```python
from build123d import *

# Parameters (mm, degrees)
SKETCH2_R           = 4.5
BOSS_EXTRUDE1_DEPTH = 76
SKETCH3_W           = 19
SKETCH3_H           = 19
BOSS_EXTRUDE2_DEPTH = 6
CHAMFER1_SIZE       = 1
CHAMFER1_SIZE2      = 1.732050808
SKETCH4_OUTSIDE_W   = 50.258
SKETCH4_OUTSIDE_H   = 50.258
SKETCH4_OUTSIDE_R   = 9.5
CUT_EXTRUDE1_DEPTH  = 6
CUT_EXTRUDE1_DRAFT  = -45


with BuildPart() as part:
    # Sketch2 → Boss-Extrude1 (new body)
    with BuildSketch(Plane.XY):
        Circle(SKETCH2_R)
    extrude(amount=BOSS_EXTRUDE1_DEPTH)

    # Sketch3 → Boss-Extrude2 (add)
    with BuildSketch(Plane.XY.offset(76)):
        Rectangle(SKETCH3_W, SKETCH3_H)
    extrude(amount=BOSS_EXTRUDE2_DEPTH)

    # Chamfer1
    chamfer1_edges = [part.edges().sort_by_distance(p)[0] for p in [
        (-4.5, 0, 0),
    ]]
    chamfer1_side = [part.faces().sort_by_distance(p)[0] for p in [
        (0, 0, 0),
    ]]
    chamfer(chamfer1_edges, length=CHAMFER1_SIZE, length2=CHAMFER1_SIZE2, reference=chamfer1_side[0])


with BuildPart() as cut_extrude1_tool:
    # Sketch4 outside → Cut-Extrude1 (with draft: the straight prism first)
    with BuildSketch(Plane.XY.offset(82)):
        Rectangle(SKETCH4_OUTSIDE_W, SKETCH4_OUTSIDE_H)
        Circle(SKETCH4_OUTSIDE_R, mode=Mode.SUBTRACT)
    extrude(amount=-CUT_EXTRUDE1_DEPTH)
    # Cut-Extrude1: the draft: its side faces are tilted about the plane it starts from
    cut_extrude1_sides = [cut_extrude1_tool.faces().sort_by_distance(p)[0] for p in [
        (0, -25.129, 79),
        (25.129, 0, 79),
        (0, 25.129, 79),
        (-25.129, 0, 79),
        (-9.5, 0, 79),
    ]]
    draft(cut_extrude1_sides, Plane.XY.offset(82), CUT_EXTRUDE1_DRAFT)


with BuildPart() as part_1:
    add(part.part)

    # Cut-Extrude1: cut by cut_extrude1_tool
    add(cut_extrude1_tool.part, mode=Mode.SUBTRACT)


solid = part_1.part
```
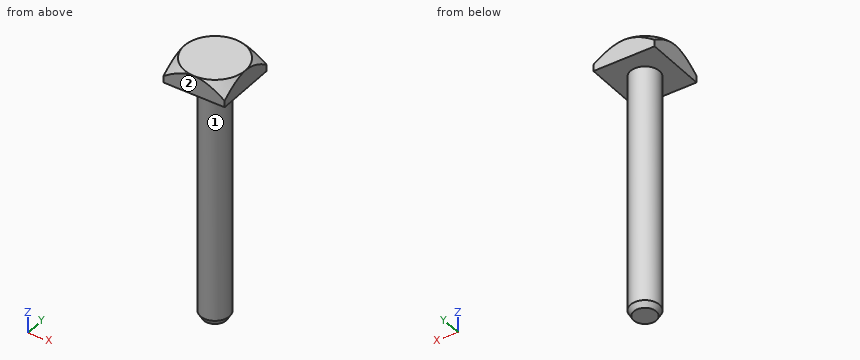
The model under review builds one solid part; all positions refer to its coordinate system, in mm. Face numbers are marked on the shaded views. A direction names the side the tool comes from. Round coordinates to 2 decimals unless told otherwise and drop trailing zeros. Write each loop counter-clockwise with the first axis right and the second up, starting at its lowest first coordinate (ties: lowest second). Pieces come first, ordered by that corner, then holes. Notation, with made-up numbers: (55.25, -18.5) -> (60.25, -18.5) arc R25 cw to (60.25, 8.5) -> close; hole circle Ø9 at (45, 45.25). An arc over 180 degrees is marked (long way). Use CSV: the item, a comma, the result in double quotes.
Q1. To check wall thickness, follow probe 1 along Z at (x, y) = (6.25, 5.25); probe 2 along Y at (x, z) = (2.5, 75.5); probe 3 along Z at (x, y) = (8.25, -8). State the ranges of each line that lie inside material, in increasing order. Write a range as [from, to].
Checks:
probe 1,"[76, 82]"
probe 2,"[-3.74, 3.74]"
probe 3,"[76, 80.01]"
Q2. For pin 1 Ø5 at (x, y) = (6, 5) entering from -Z; pin 2 Ø8 at (y, z) = (5, 57) entering from -X; pin 3 Ø10 at (x, z) = (6.5, 71.5) entering from +Y; pin 4 Ø3 at (y, z) = (2, 32) entering from -X, all flat-tipped, find the tip position at first contact; note any pin that passes through.
Checks:
pin 1,"z = 76"
pin 2,"x = -4.39"
pin 3,"y = 9.5"
pin 4,"x = -4.47"
Q3. For the marked faces 1 and 2, list the 3-axis set-ups (+Z, -Z, +X, -X, +Y, -Y) from which the entire face can be reached by the end or side of a thin tool; tool diameter is ignored.
Checks:
face 1,"-Z"
face 2,"+Z, -Z, +X, -X, -Y"
Q4. Consider section A-A (z = 29.5). Give the boundary of the cut face in (x, y), then the cut area to 3 significant figures.
Checks:
outline,"circle Ø9 at (0, 0)"
area,"63.6 mm²"
